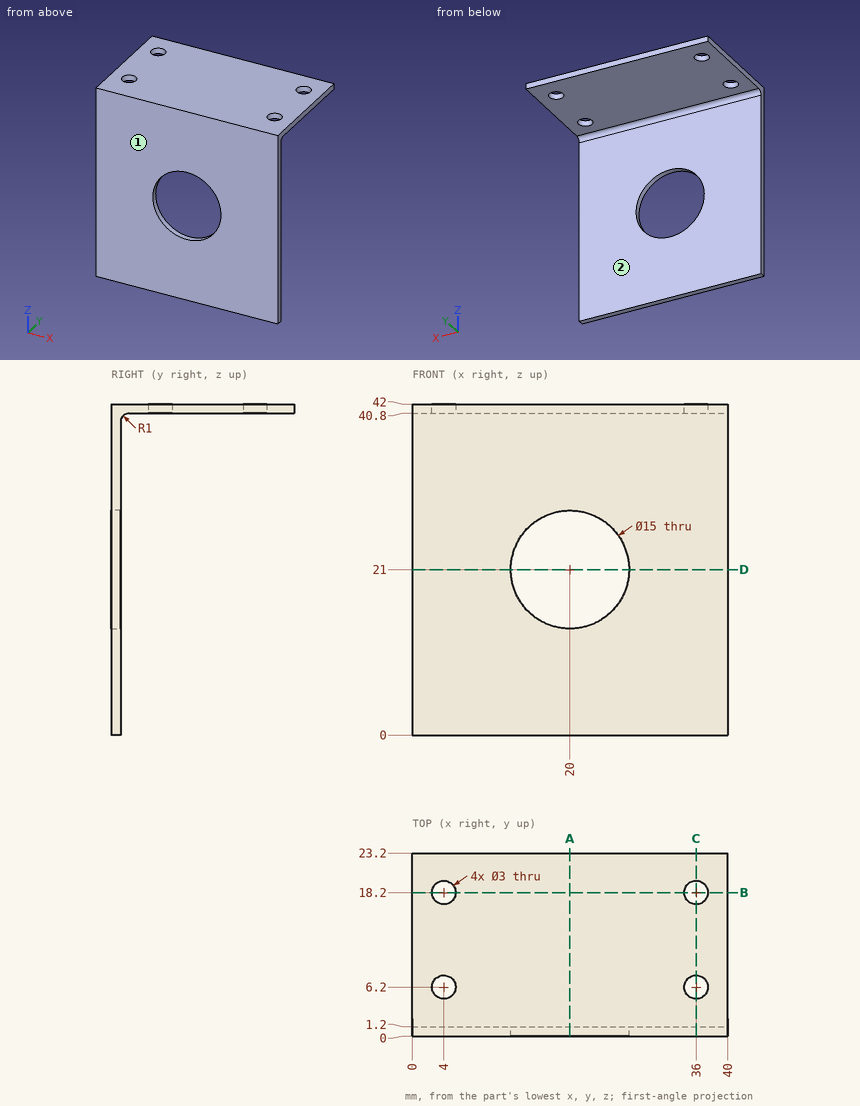
Design review of the part shown in the three views and the two pictorial views. Dimensions are in mm from the part's minimum x, y and z. A direction names the side the tool comes from. Round coordinates to 2 decimals unless told otherwise and drop trailing zeros. Loops run counter-clockwise (first coordinate to the right, second up) from the corner with the lowest first, then second, coordinate; pieces in that order, holes last. Notation, with made-up numbers: M 78.25,17 L 84.25,17 A15 ccw 84.25,45 Z; hole C 5.25,59.5 d3. An arc over 180 degrees is marked long. Put each result on its own line as item: value.
Q1. Consider section B-B, the plane y = 18.2. Give the boundary of the cut face in (x, z), then the cut area to 3 significant figures.
Result set:
outline: M 0,40.8 L 2.5,40.8 L 2.5,42 L 0,42 Z; M 5.5,40.8 L 34.5,40.8 L 34.5,42 L 5.5,42 Z; M 37.5,40.8 L 40,40.8 L 40,42 L 37.5,42 Z
area: 40.8 mm²
Q2. Consider section C-C, the plane x = 36. Give the boundary of the cut face in (y, z).
Result set:
outline: M 0,0 L 1.2,0 L 1.2,39.8 A1 cw 2.2,40.8 L 4.7,40.8 L 4.7,42 L 0,42 Z; M 7.7,40.8 L 16.7,40.8 L 16.7,42 L 7.7,42 Z; M 19.7,40.8 L 23.2,40.8 L 23.2,42 L 19.7,42 Z
Q3. For pin 1 (10 mm diameter, centred on x = 8, z = 17.5, fed in from +Y); pin 2 (4 mm diameter, centred on x = 36, y = 18.2, fed in from -Z), all flat-tipped, find the tip position at first contact; note any pin that passes through.
Result set:
pin 1: stops at y = 1.2
pin 2: stops at z = 40.8
Q4. Consider section A-A, the plane x = 20. Give the boundary of the cut face in (y, z).
Result set:
outline: M 0,0 L 1.2,0 L 1.2,13.5 L 0,13.5 Z; M 0,28.5 L 1.2,28.5 L 1.2,39.8 A1 cw 2.2,40.8 L 23.2,40.8 L 23.2,42 L 0,42 Z
Q5. To check wall thickness, follow L1, parallel to Y at x = 36, z = 41.15; L2, parallel to X at y = 0.6, z = 21; L3, parallel to Z at x = 27, y = 17.5. State the ranges of each line that lie inside material, in increasing order.
Result set:
L1: y = 0 to 4.7, 7.7 to 16.7, 19.7 to 23.2
L2: x = 0 to 12.5, 27.5 to 40
L3: z = 40.8 to 42
Q6. Consider section D-D, the plane z = 21. Give the boundary of the cut face in (x, y).
Result set:
outline: M 0,0 L 12.5,0 L 12.5,1.2 L 0,1.2 Z; M 27.5,0 L 40,0 L 40,1.2 L 27.5,1.2 Z
Q7. Machinability: for the marked faces 1 and 2, which of the approach directions +Z, -Z, +X, -X, +Y, -Y give a long, thin tool a straight path to every point of the face, cutting with its end or side? Answer none if there is none.
Result set:
face 1: +Z, -Z, +X, -X, -Y
face 2: -Z, +X, -X, +Y
